Check sheet for the modelled part. Datum: model origin and axes. Units: mm. A direction names the side the tool comes from. Coordinates: 2 decimals unless noted, no trailing zeros. Loops run counter-clockwise (first coordinate to the right, second up) from the corner with the lowest first, then second, coordinate; pieces in that order, holes last. Notation, with made-up numbers: M 5,-38.5 L 62,-38.5 A16 ccw 62,-19.5 Z; hole C 86,47 d6. An arc over 180 degrees is marked long. Return JSON: item names as keys, results as strings.
from build123d import *

# Parameters (mm, degrees)
SKETCH1_R           = 12.5
SKETCH1_R_2         = 3.425
BOSS_EXTRUDE1_DEPTH = 10
SKETCH2_W           = 5
SKETCH2_H           = 5
CHAMFER1_SIZE       = 0.5
FILLET1_R           = 0.5


with BuildPart() as part:
    # Sketch1 → Boss-Extrude1 (new body)
    with BuildSketch(Plane.XY):
        Circle(SKETCH1_R)
        Circle(SKETCH1_R_2, mode=Mode.SUBTRACT)
    extrude(amount=BOSS_EXTRUDE1_DEPTH)

    # Sketch2 → Cut-Revolve1 (revolve, cut)
    with BuildSketch(Plane(origin=(0, 0, 0), x_dir=(1, 0, 0), z_dir=(0, 1, 0))):
        with Locations((-10, -5)):
            Rectangle(SKETCH2_W, SKETCH2_H)
    revolve(axis=Axis((0, 0, 0), (0, 0, 1)), mode=Mode.SUBTRACT)

    # Chamfer1
    chamfer1_edges = [part.edges().sort_by_distance(p)[0] for p in [
        (-12.5, 0, 2.5),
        (-12.5, 0, 7.5),
        (-12.5, 0, 10),
        (-12.5, 0, 0),
        (-3.425, 0, 0),
        (-3.425, 0, 10),
    ]]
    chamfer(chamfer1_edges, length=CHAMFER1_SIZE)

    # Fillet1
    fillet1_edges = [part.edges().sort_by_distance(p)[0] for p in [
        (7.5, 0, 7.5),
        (7.5, 0, 2.5),
    ]]
    fillet(fillet1_edges, radius=FILLET1_R)


solid = part.part
1) Section check C-C on z = 3.5. Record the cut outline in (x, y) (3 decimals).
Answers:
{"outline": "C 0,0 d15; hole C 0,0 d6.85"}
2) Draft check along Z on faces 3 (the face through (-2, 8, 2.5)), 4 (the face through (-3, 3, 0)), 5 (the face through (11.923, 3.755, 8.74)). Enter one of: +Z half, -Z half, draft (parallel to the pull), parting line (faces both ways), or undercut.
Answers:
{"face 3": "undercut", "face 4": "-Z half", "face 5": "draft"}
3) Scan lines: line 1 along Y through (x, z) = (0, 5.5) (3 decimals); line 2 along Z through (x, y) = (6.75, 4.5); line 3 along Y through (x, z) = (2.75, 8.5). Record each from-to range of solid material in increasing order. Write a range as [from, to].
Answers:
{"line 1": "[-7.5, -3.425], [3.425, 7.5]", "line 2": "[0, 2.5], [7.5, 10]", "line 3": "[-12.19, -2.04], [2.04, 12.19]"}
4) Set-up check for faces 1 (the face through (7.493, -0.33, 4.972)), 2 (the face through (-3, 3, 10)): record each of +Z, -Z, +X, -X, +Y, -Y from which the full face is reachable in a straight line by a thin tool's end or side.
Answers:
{"face 1": "none", "face 2": "+Z, +X, -X, +Y, -Y"}
5) Go/stop test with flat-tipped pins: pin 1 Ø2 at (y, z) = (4.5, 4.5) entering from +X; pin 2 Ø5 at (y, z) = (-9.5, 3) entering from +X; pin 3 Ø5 at (x, z) = (-7, 3.5) entering from +Y. Record where each tip stops, or that it passes through.
Answers:
{"pin 1": "x = 6.63", "pin 2": "x = 10.21", "pin 3": "y = 11.46"}
